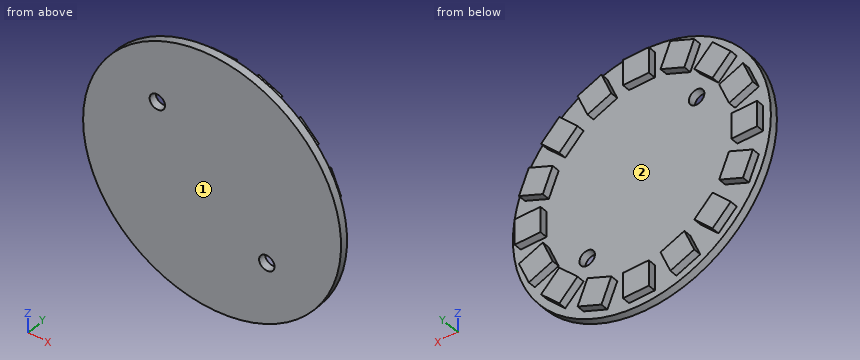
Autodesk Inventor part; units mm, degrees
ref_plane "YZ Plane" through (0, 0, 0) normal (1, 0, 0) x (0, 1, 0)
ref_plane "XZ Plane" through (0, 0, 0) normal (0, 1, 0) x (-1, 0, 0)
ref_plane "XY Plane" through (0, 0, 0) normal (0, 0, 1) x (1, 0, 0)
sketch "Sketch1" plane through (0, 0, 0) normal (0, 1, 0) x (-1, 0, 0)
  circle A0 centre (0, 0) radius 25
  line L0 (0, 0) -> (10.6066, 10.6066)
  line L1 (0, 0) -> (15, 0) construction
  circle A1 centre (10.6066, 10.6066) radius 1.5
  line L2 (0, 0) -> (-10.6066, -10.6066)
  line L3 (0, 0) -> (15, 0) construction
  circle A2 centre (-10.6066, -10.6066) radius 1.5
  dimension "d0" = 50
  dimension "d1" = 15
  dimension "d2" = 45
  dimension "d3" = 3
  dimension "d4" = 15
  dimension "d5" = 135
  dimension "d6" = 3
extrude "Extrusion1" add sketch "Sketch1" along normal blind 1.5
sketch "Sketch2" plane through (0, 1.5, 0) normal (0, 1, 0) x (1, 0, 0)
  line L0 (0, 0) -> (-23.5, 0)
  line L1 (0, 0) -> (23.5, 0) construction
  line L2 (-23.5, 0) -> (-23.5, 2.5)
  line L3 (-23.5, 2.5) -> (-18.5, 2.5)
  line L4 (-18.5, 2.5) -> (-18.5, -2.5)
  line L5 (-18.5, -2.5) -> (-23.5, -2.5)
  line L6 (-23.5, -2.5) -> (-23.5, 2.5)
  dimension "d9" = 23.5
  dimension "d10" = 180
  dimension "d11" = 2.5
  dimension "d12" = 90
  dimension "d13" = 5
  dimension "d14" = 5
extrude "Extrusion2" add sketch "Sketch2" along normal blind 1.5
pattern_circular "Circular Pattern1" count 16 over 360 about axis through (0, 0, 0) along (0, 1, 0) of "Extrusion2"
properties part number "WifiPixels"
Part model, mm, in its own coordinate system. Face numbers are marked on the shaded views. Give positions to 0.01 mm unless a question says otherwise; leave off trailing zeros. Write each loop counter-clockwise with the first axis right and the second up, starting at its lowest first coordinate (ties: lowest second). Pieces come first, ordered by that corner, then holes. Notation, with made-up numbers: M 34.25,83.5 L 56.25,83.5 A12 cw 56.25,87.5 Z; hole C 58.25,53 d2. An arc over 180 degrees is marked long. Use CSV: the item, a comma, the result in double quotes.
Item 1: Slice it at C-C on y = 2.05. State how many separate pieces and enclosed holes the cut face has, plus the area to 3 significant figures.
Taken from the geometry:
separate pieces,"16"
enclosed holes,"0"
area,"400 mm²"
Item 2: Pull direction Z, two halves, no side cores. Call the marked faces 1 and 2: +Z half, -Z half, draft (parallel to the pull), parting line (faces both ways), or undercut.
Taken from the geometry:
face 1,"draft"
face 2,"undercut"
Item 3: Drill centre lines: probe 1 along Z at (x, y) = (-1, 2.25); probe 2 along X at (y, z) = (2.4, -21). Where is each one in solid material? Low to high.
Taken from the geometry:
probe 1,"z = -23.5 to -18.5, 18.5 to 23.5"
probe 2,"x = -10.71 to -5.99, -2.5 to 2.5, 5.99 to 10.71"
Item 4: Pin check, flat tips, straight feed: P1, Ø1.2, axis at x = -0.5, y = 2, coming from the -Z side; P2, Ø2, axis at x = 14, z = 8.5, coming from the +Y side; P3, Ø0.8, axis at x = -20, y = 2.5, coming from the +Z side. Stop position of each tip, or through.
Taken from the geometry:
P1,"stops at z = -25"
P2,"stops at y = 1.5"
P3,"stops at z = 11.16"
Item 5: Slice it at B-B on x = 0. Write the cut outline in (y, z).
Taken from the geometry:
outline,"M 0,-25 L 1.5,-25 L 1.5,-23.5 L 3,-23.5 L 3,-18.5 L 1.5,-18.5 L 1.5,18.5 L 3,18.5 L 3,23.5 L 1.5,23.5 L 1.5,25 L 0,25 Z"
Item 6: Slice it at A-A on z = 0. Write the cut outline in (x, y), plus the area to 3 significant figures.
Taken from the geometry:
outline,"M -25,0 L 25,0 L 25,1.5 L 23.5,1.5 L 23.5,3 L 18.5,3 L 18.5,1.5 L -18.5,1.5 L -18.5,3 L -23.5,3 L -23.5,1.5 L -25,1.5 Z"
area,"90.0 mm²"
